```python
from build123d import *

# Parameters (mm, degrees)
SKETCH1_W                 = 130
SKETCH1_H                 = 125
BOSS_EXTRUDE1_DEPTH       = 5
SKETCH2_R                 = 1.75
SKETCH2_R_2               = 12.65
CUT_EXTRUDE1_DEPTH        = 10
SKETCH4_R                 = 2.15
CUT_EXTRUDE3_DEPTH        = 10
BOSS_EXTRUDE2_DEPTH       = 2
MIRROR7_COPY_1_SKETCH_R   = 1.75
MIRROR7_COPY_1_SKETCH_R_2 = 12.65
MIRROR7_COPY_1_DEPTH      = 10
MIRROR7_COPY_2_DEPTH      = 2
SKETCH10_R                = 2.15
CUT_EXTRUDE8_DEPTH        = 91.311959341
SKETCH11_R                = 2.65
CUT_EXTRUDE9_DEPTH        = 0.5
CUT_EXTRUDE10_DEPTH       = 91.444734507
CUT_EXTRUDE11_DEPTH       = 91.444734507
CUT_EXTRUDE12_DEPTH       = 91.444734507


with BuildPart() as part:
    # Sketch1 → Boss-Extrude1 (new body)
    with BuildSketch(Plane(origin=(0, 0, 0), x_dir=(1, 0, 0), z_dir=(0, 1, 0))):
        Rectangle(SKETCH1_W, SKETCH1_H)
    extrude(amount=BOSS_EXTRUDE1_DEPTH)

    # Sketch2 → Cut-Extrude1 (cut)
    with BuildSketch(Plane(origin=(0, 5, 0), x_dir=(1, 0, 0), z_dir=(0, 1, 0))):
        with Locations(Location((-61, -52.5, 0), (0, 0, 270))):
            Circle(SKETCH2_R)
        with Locations(Location((-36, -52.5, 0), (0, 0, 270))):
            Circle(SKETCH2_R)
        with Locations(Location((-36, -10.5, 0), (0, 0, 270))):
            Circle(SKETCH2_R)
        with Locations(Location((-61, -10.5, 0), (0, 0, 270))):
            Circle(SKETCH2_R)
        with Locations(Location((-45.5, -31.5, 0), (0, 0, 270))):
            Circle(SKETCH2_R_2)
    cut_extrude1 = extrude(amount=-CUT_EXTRUDE1_DEPTH, mode=Mode.SUBTRACT)

    # Mirror3: Cut-Extrude1 across plane
    add(cut_extrude1.mirror(Plane.ZY), mode=Mode.SUBTRACT)

    # Sketch4 → Cut-Extrude3 (cut)
    with BuildSketch(Plane(origin=(0, 5, 0), x_dir=(1, 0, 0), z_dir=(0, 1, 0))):
        with Locations(Location((0, 47.5, 0), (0, 0, 270))):
            Circle(SKETCH4_R)
        with Locations(Location((12.049810205, 55, 0), (0, 0, 270))):
            Circle(SKETCH4_R)
        with Locations(Location((-12.049810205, 55, 0), (0, 0, 270))):
            Circle(SKETCH4_R)
    extrude(amount=-CUT_EXTRUDE3_DEPTH, mode=Mode.SUBTRACT)

    # Sketch5 → Boss-Extrude2 (add)
    with BuildSketch(Plane.XZ):
        Polygon((-65, 58.7), (-65, 56.7), (-31.6, 56.7), (-31.6, 6.3), (-65, 6.3), (-65, 4.3), (-29.6, 4.3), (-29.6, 58.7), align=None)
    boss_extrude2 = extrude(amount=BOSS_EXTRUDE2_DEPTH)

    # Mirror5: Boss-Extrude2 across plane
    add(boss_extrude2.mirror(Plane.ZY))

    # Mirror7: Cut-Extrude1, Boss-Extrude2 across plane
    add(cut_extrude1.mirror(Plane.XY.offset(-1.9)), mode=Mode.SUBTRACT)
    add(boss_extrude2.mirror(Plane.XY.offset(-1.9)))

    # Mirror7 copy 1 sketch → Mirror7 copy 1 (cut)
    with BuildSketch(Plane(origin=(0, 5, -3.8), x_dir=(-1, 0, 0), z_dir=(0, 1, 0))):
        with Locations(Location((-61, -52.5, 0), (0, 0, 270))):
            Circle(MIRROR7_COPY_1_SKETCH_R)
        with Locations(Location((-36, -52.5, 0), (0, 0, 270))):
            Circle(MIRROR7_COPY_1_SKETCH_R)
        with Locations(Location((-36, -10.5, 0), (0, 0, 270))):
            Circle(MIRROR7_COPY_1_SKETCH_R)
        with Locations(Location((-61, -10.5, 0), (0, 0, 270))):
            Circle(MIRROR7_COPY_1_SKETCH_R)
        with Locations(Location((-45.5, -31.5, 0), (0, 0, 270))):
            Circle(MIRROR7_COPY_1_SKETCH_R_2)
    extrude(amount=-MIRROR7_COPY_1_DEPTH, mode=Mode.SUBTRACT)

    # Mirror7 copy 2 sketch → Mirror7 copy 2 (add)
    with BuildSketch(Plane(origin=(0, 0, -3.8), x_dir=(-1, 0, 0), z_dir=(0, -1, 0))):
        Polygon((-65, 58.7), (-65, 56.7), (-31.6, 56.7), (-31.6, 6.3), (-65, 6.3), (-65, 4.3), (-29.6, 4.3), (-29.6, 58.7), align=None)
    extrude(amount=MIRROR7_COPY_2_DEPTH)

    # Sketch10 → Cut-Extrude8 (cut, through all)
    with BuildSketch(Plane(origin=(0, 0, 0), x_dir=(-1, 0, 0), z_dir=(0, -1, 0))):
        with Locations(Location((-24.17, -42.03, 0), (0, 0, 90))):
            Circle(SKETCH10_R)
        with Locations(Location((24.17, -42.03, 0), (0, 0, 90))):
            Circle(SKETCH10_R)
        with Locations(Location((-8.73, 9.6, 0), (0, 0, 90))):
            Circle(SKETCH10_R)
        with Locations(Location((19.29, 9.6, 0), (0, 0, 90))):
            Circle(SKETCH10_R)
        with Locations(Location((-24.17, 33.11, 0), (0, 0, 90))):
            Circle(SKETCH10_R)
        with Locations(Location((24.17, 40.6, 0), (0, 0, 90))):
            Circle(SKETCH10_R)
    extrude(amount=-CUT_EXTRUDE8_DEPTH, mode=Mode.SUBTRACT)

    # Sketch11 → Cut-Extrude9 (cut)
    with BuildSketch(Plane.XZ):
        with Locations(Location((-12.049810205, -55, 0), (0, 0, 270))):
            Circle(SKETCH11_R)
        with Locations(Location((0, -47.5, 0), (0, 0, 270))):
            Circle(SKETCH11_R)
        with Locations(Location((12.049810205, -55, 0), (0, 0, 270))):
            Circle(SKETCH11_R)
        with Locations(Location((-24.17, -40.6, 0), (0, 0, 270))):
            Circle(SKETCH11_R)
        with Locations(Location((24.17, -33.11, 0), (0, 0, 270))):
            Circle(SKETCH11_R)
        with Locations(Location((8.73, -9.6, 0), (0, 0, 270))):
            Circle(SKETCH11_R)
        with Locations(Location((-19.29, -9.6, 0), (0, 0, 270))):
            Circle(SKETCH11_R)
        with Locations(Location((-24.17, 42.03, 0), (0, 0, 270))):
            Circle(SKETCH11_R)
        with Locations(Location((24.17, 42.03, 0), (0, 0, 270))):
            Circle(SKETCH11_R)
        with Locations(Location((-61, -14.3, 0), (0, 0, 270))):
            Circle(SKETCH11_R)
        with Locations(Location((-36, -14.3, 0), (0, 0, 270))):
            Circle(SKETCH11_R)
        with Locations(Location((-61, -56.3, 0), (0, 0, 270))):
            Circle(SKETCH11_R)
        with Locations(Location((-36, -56.3, 0), (0, 0, 270))):
            Circle(SKETCH11_R)
        with Locations(Location((36, -56.3, 0), (0, 0, 270))):
            Circle(SKETCH11_R)
        with Locations(Location((61, -56.3, 0), (0, 0, 270))):
            Circle(SKETCH11_R)
        with Locations(Location((36, -14.3, 0), (0, 0, 270))):
            Circle(SKETCH11_R)
        with Locations(Location((61, -14.3, 0), (0, 0, 270))):
            Circle(SKETCH11_R)
        with Locations(Location((36, 10.5, 0), (0, 0, 270))):
            Circle(SKETCH11_R)
        with Locations(Location((61, 10.5, 0), (0, 0, 270))):
            Circle(SKETCH11_R)
        with Locations(Location((61, 52.5, 0), (0, 0, 270))):
            Circle(SKETCH11_R)
        with Locations(Location((36, 52.5, 0), (0, 0, 270))):
            Circle(SKETCH11_R)
        with Locations(Location((-36, 52.5, 0), (0, 0, 270))):
            Circle(SKETCH11_R)
        with Locations(Location((-36, 10.5, 0), (0, 0, 270))):
            Circle(SKETCH11_R)
        with Locations(Location((-61, 10.5, 0), (0, 0, 270))):
            Circle(SKETCH11_R)
        with Locations(Location((-61, 52.5, 0), (0, 0, 270))):
            Circle(SKETCH11_R)
    extrude(amount=-CUT_EXTRUDE9_DEPTH, mode=Mode.SUBTRACT)

    # Sketch12 → Cut-Extrude10 (cut, through all)
    with BuildSketch(Plane(origin=(0, 5, 0), x_dir=(1, 0, 0), z_dir=(0, 1, 0))):
        Polygon((-2.363095604, -26.45), (-20.17, 1.845056316), (-20.17, -54.745056316), align=None)
        Polygon((17.806904396, 5.6), (-17.806904396, 5.6), (0, -22.695056316), align=None)
        Polygon((20.17, -54.745056316), (20.17, 1.845056316), (2.363095604, -26.45), align=None)
        Polygon((0, -30.204943684), (-17.806904396, -58.5), (17.806904396, -58.5), align=None)
    extrude(amount=-CUT_EXTRUDE10_DEPTH, mode=Mode.SUBTRACT)

    # Sketch13 → Cut-Extrude11 (cut, through all)
    with BuildSketch(Plane(origin=(0, 5, 0), x_dir=(1, 0, 0), z_dir=(0, 1, 0))):
        Polygon((-61, 1.9), (-61, -3.1), (-24.17, -3.1), (-24.17, 6.9), (-61, 6.9), align=None)
    cut_extrude11 = extrude(amount=-CUT_EXTRUDE11_DEPTH, mode=Mode.SUBTRACT)

    # Mirror9: Cut-Extrude11 across plane
    add(cut_extrude11.mirror(Plane.ZY), mode=Mode.SUBTRACT)

    # Sketch14 → Cut-Extrude12 (cut, through all)
    with BuildSketch(Plane(origin=(0, 5, 0), x_dir=(1, 0, 0), z_dir=(0, 1, 0))):
        Polygon((-3.110442245, 28.55), (-17.806904396, 40.888590935), (-17.806904396, 16.211409065), align=None)
        Polygon((14.696462151, 43.5), (-14.696462151, 43.5), (0, 31.161409065), align=None)
        Polygon((17.806904396, 16.211409065), (17.806904396, 40.888590935), (3.110442245, 28.55), align=None)
        Polygon((0, 25.938590935), (-14.696462151, 13.6), (14.696462151, 13.6), align=None)
    extrude(amount=-CUT_EXTRUDE12_DEPTH, mode=Mode.SUBTRACT)


solid = part.part
```
CAD build for the part. Positions are in the model's coordinates, mm. A direction names the side the tool comes from. Coordinates: 2 decimals unless noted, no trailing zeros. Order: outer loops, then holes, each group sorted by start corner. A loop starts at its lowest first (then second) coordinate and runs counter-clockwise, first axis right, second up. Notation, with made-up numbers: (85.5, 76) - (121.5, 76) arc R17 ccw to (121.5, 105) - close; hole circle Ø1 at (-27.75, 51). An arc over 180 degrees is marked (long way). Use a Markdown table: item, result. Add a question column.
(1) Saw through at A-A (x = 45.5). Count the separate pieces of the cut face and the enclosed holes in it, then the cut area to 3 significant figures.
(2) Drill centre lines: line 1 along X through (y, z) = (-1.5, -14); line 2 along X through (y, z) = (2.5, 28); line 3 along X through (y, z) = (3, -8.5). Where is each one in solid material? Low to high. Write a range as [from, to].
(3) Saw through at B-B (z = 47.5). Give the cut face in (x, y).
(4) Which spindle directions (+Z, -Z, +X, -X, +Y, -Y) get a long thin tool onto all of the face, cutting with end or side? Do faces 1 (the face through (43, 3, 3.1)), 2 (the face through (-63.351, 0.246, -15.523)). Say none if no direction does.
(5) Pull direction X, two halves, no side cores. Call faces 3 (the face through (-63, 0.5, 10)), 4 (the face through (30, -2, -35)), 5 (the face through (34, 0.5, 10)): +X half, -X half, draft (parallel to the pull), parting line (faces both ways), or undercut.
(6) Flat gauge pins, fed straight in: pin 1 (16.5 mm diameter, centred on x = 49.5, z = -31.5, fed in from -Y); pin 2 (1.6 mm diameter, centred on x = -20.5, z = -10.5, fed in from -Y); pin 3 (1.6 mm diameter, centred on x = 45.5, y = -1, fed in from +Z). Where does each tip first touch, or does it go through?
Solved:
| question | item | result |
|---|---|---|
| 1 | separate pieces | 4 |
| 1 | enclosed holes | 0 |
| 1 | area | 338 mm² |
| 2 | line 1 | x = [-31.6, -29.6], [29.6, 31.6] |
| 2 | line 2 | x = [-65, -57.66], [-33.34, -20.17], [-3.34, 3.34], [20.17, 33.34], [57.66, 65] |
| 2 | line 3 | x = [-65, -21.14], [-17.44, 6.88], [10.58, 65] |
| 3 | outline | (-65, 0) - (-31.6, 0) - (-31.6, -2) - (-29.6, -2) - (-29.6, 0) - (-20.17, 0) - (-20.17, 5) - (-65, 5) - close; (-15.61, 0) - (-10.88, 0) - (-10.88, 5) - (-15.61, 5) - close; (10.88, 0) - (15.61, 0) - (15.61, 5) - (10.88, 5) - close; (20.17, 0) - (29.6, 0) - (29.6, -2) - (31.6, -2) - (31.6, 0) - (65, 0) - (65, 5) - (20.17, 5) - close |
| 4 | face 1 | +Y, -Y |
| 4 | face 2 | -Y |
| 5 | face 3 | undercut |
| 5 | face 4 | draft |
| 5 | face 5 | undercut |
| 6 | pin 1 | stops at y = 0 |
| 6 | pin 2 | stops at y = 0.5 |
| 6 | pin 3 | stops at z = 58.7 |
